Check sheet for the drawn part. Datum: minimum x, y, z corner. Units: mm. A direction names the side the tool comes from. Round coordinates to 2 decimals unless told otherwise and drop trailing zeros. Order: outer loops, then holes, each group sorted by start corner. A loop starts at its lowest first (then second) coordinate and runs counter-clockwise, first axis right, second up.
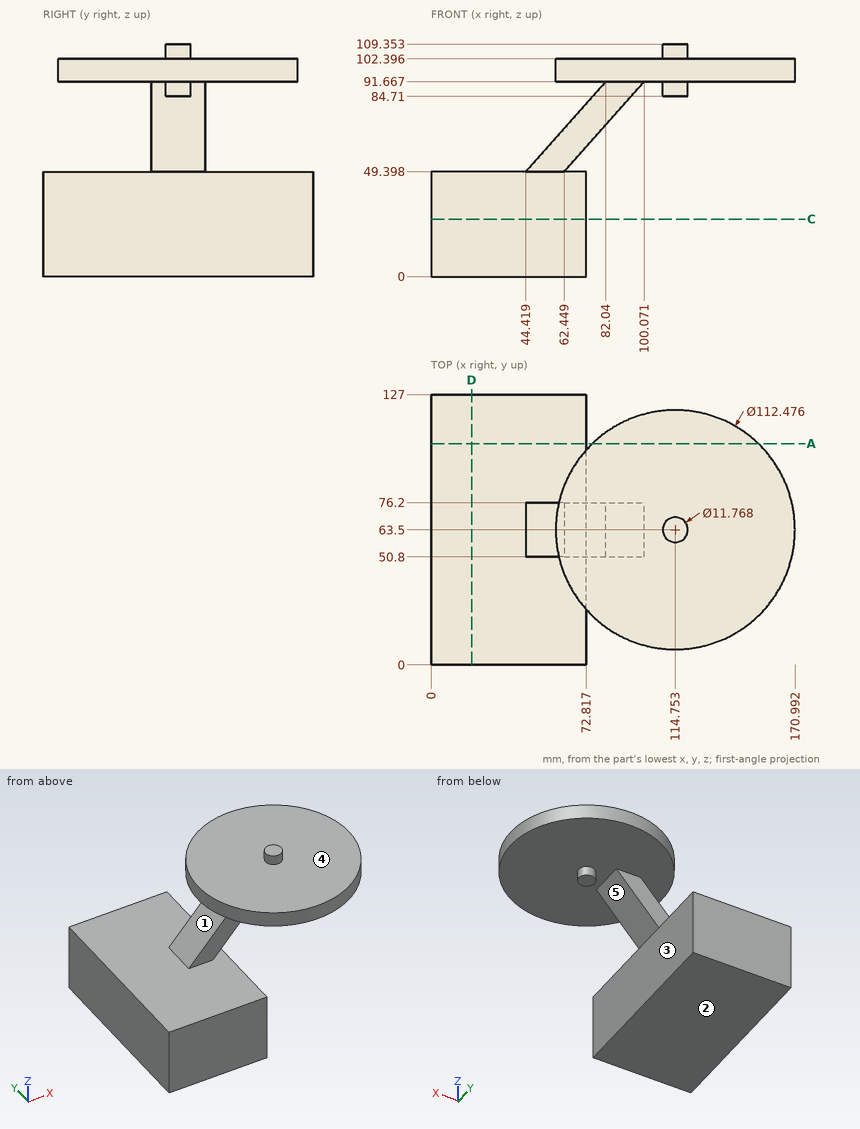
(1) Sectioned sample at C-C, the plane z = 27. Record the cut outline in (x, y), and give its area (3 significant figures).
Returned:
outline: (0, 0) - (72.82, 0) - (72.82, 127) - (0, 127) - close
area: 9,250 mm2
(2) Set-up check for the marked faces 1 and 2: record each of +Z, -Z, +X, -X, +Y, -Y from which the full face is reachable in a straight line by a thin tool's end or side.
Returned:
face 1: -X, +Y, -Y
face 2: -Z, +X, -X, +Y, -Y
(3) Sectioned sample at A-A, the plane y = 104. Record the cut outline in (x, z) (1 decimal).
Returned:
outline: (0, 0) - (72.8, 0) - (72.8, 49.4) - (0, 49.4) - close; (75.7, 91.7) - (153.8, 91.7) - (153.8, 102.4) - (75.7, 102.4) - close
(4) Depth check by flat-ended pin: P1, Ø4, axis at x = 87.5, y = 102.5, coming from the -Z side; P2, Ø6, axis at y = 50.5, z = 15, coming from the -X side; P3, Ø8, axis at x = 48, y = 89, coming from the +Z side; P4, Ø12.5, axis at x = 70, z = 71.5, coming from the +Y side. Enter the tip coordinate at first touch or a pass-through.
Returned:
P1: stops at z = 91.67
P2: stops at x = 0
P3: stops at z = 49.4
P4: stops at y = 76.2
(5) Sectioned sample at D-D, the plane x = 19. Record the cut outline in (y, z), and give its area (3 significant figures).
Returned:
outline: (0, 0) - (127, 0) - (127, 49.4) - (0, 49.4) - close
area: 6,270 mm2
(6) Draft check along Z on the marked faces 3, 4 and 5. Enter one of: released by +Z, released by -Z, zero draft, split by the parting line, or undercut.
Returned:
face 3: zero draft
face 4: released by +Z
face 5: undercut
(7) Material ranges on line 1 (Z direction, x = 69.5, y = 82); line 2 (Y direction, x = 49, z = 53.5); line 3 (Z direction, x = 63.5, y = 51) (1 decimal), recorded low to high.
Returned:
line 1: z = 0 to 49.4, 91.67 to 102.4
line 2: y = 50.8 to 76.2
line 3: z = 0 to 49.4, 50.6 to 70.8, 91.7 to 102.4
